Design review of the part built by this model. Coordinates are the model's own, in mm. A direction names the side the tool comes from. Give positions to 0.01 mm unless a question says otherwise; leave off trailing zeros. Order: outer loops, then holes, each group sorted by start corner. A loop starts at its lowest first (then second) coordinate and runs counter-clockwise, first axis right, second up.
Autodesk Inventor part; units mm, degrees
ref_plane "工作平面1" through (0, 0, 5.8) normal (0, 0, 1) x (1, 0, 0)
ref_plane "YZ Plane" through (0, 0, 0) normal (1, 0, 0) x (0, 1, 0)
ref_plane "XZ Plane" through (0, 0, 0) normal (0, 1, 0) x (-1, 0, 0)
sketch "草圖1" plane through (0, 0, 0) normal (0, 0, 1) x (1, 0, 0)
  circle A0 centre (0, 0) radius 26
  dimension "d0" = 52
extrude "擠出1" add sketch "草圖1" along normal blind 12.2
sketch "草圖2" plane through (0, 0, 12.2) normal (0, 0, 1) x (1, 0, 0)
  circle A0 centre (0, 0) radius 26
  circle A1 centre (0, 0) radius 20
  dimension "d3" = 40
extrude "擠出2" cut sketch "草圖2" against normal through all contours A1
sketch "草圖3" plane through (0, 0, 0) normal (0, 0, -1) x (-1, 0, 0)
  circle A0 centre (0, 0) radius 20
  circle A1 centre (0, 0) radius 26
  circle A2 centre (0, 0) radius 22.45
  dimension "d6" = 44.9
extrude "擠出3" cut sketch "草圖3" against normal blind 8.2 contours A2
ref_plane "工作平面1" through (0, 0, 5.8) normal (0, 0, 1) x (1, 0, 0)
sketch "草圖4" plane through (0, 0, 5.8) normal (0, 0, 1) x (1, 0, 0)
  circle A0 centre (0, 0) radius 24.4
  circle A1 centre (0, 0) radius 26
  dimension "d10" = 48.8
extrude "擠出4" cut sketch "草圖4" against normal blind 2.8
chamfer "倒角1" distance 0.4 angle 45 3 edges at (-26, 0, 12.2) (-26, 0, 0) (22.45, 0, 0)
chamfer "倒角2" distance 0.3 angle 45 1 edges at (-20, 0, 8.2)
properties part number "鑄鐵SLEEVE"
1. Take a section at A-A (y = 0). State the section outline as (x, z) points, then the cut area to 3 significant figures.
Recorded:
outline: (-26, 0.4) - (-25.6, 0) - (-22.85, 0) - (-22.45, 0.4) - (-22.45, 8.2) - (-20.3, 8.2) - (-20, 8.5) - (-20, 12.2) - (-25.6, 12.2) - (-26, 11.8) - (-26, 5.8) - (-24.4, 5.8) - (-24.4, 3) - (-26, 3) - close; (20, 8.5) - (20.3, 8.2) - (22.45, 8.2) - (22.45, 0.4) - (22.85, 0) - (25.6, 0) - (26, 0.4) - (26, 3) - (24.4, 3) - (24.4, 5.8) - (26, 5.8) - (26, 11.8) - (25.6, 12.2) - (20, 12.2) - close
area: 96.7 mm2
2. Take a section at D-D (z = 11). State the section outline as (x, y) points.
Recorded:
outline: circle Ø52 at (0, 0); hole circle Ø40 at (0, 0)
3. Machinability: for faces 1 (the face through (-20.633, 15.821, 8.758)), 2 (the face through (17, -12, 8.2)), which of the approach directions +Z, -Z, +X, -X, +Y, -Y give a long, thin tool a straight path to every point of the face, cutting with its end or side? Answer none if there is none.
Recorded:
face 1: +Z, -Z
face 2: -Z
4. For pin 1 (5 mm diameter, centred on y = -7.5, z = 4.5, fed in from +X); pin 2 (1.5 mm diameter, centred on y = 10, z = 4.5, fed in from +X); pin 3 (3 mm diameter, centred on x = 2.5, z = 8, fed in from -Y); pin 4 (15.5 mm diameter, centred on x = 9, y = -4, fed in from +Z), all flat-tipped, find the tip position at first contact; note any pin that passes through.
Recorded:
pin 1: stops at x = 25.44
pin 2: stops at x = 22.58
pin 3: stops at y = -25.98
pin 4: passes through
5. Draft analysis for pull direction Z (two halves, no side actions). For faces 3 (the face through (-15.3, 17.2, 0)), 4 (the face through (-4.336, -19.524, 10.376)), 5 (the face through (-24.376, 1.073, 4.42)), state which applies: pulls with the +Z half, pulls with the -Z half, needs draft (parallel to the pull), parting line crosses it, or undercut.
Recorded:
face 3: pulls with the -Z half
face 4: needs draft
face 5: undercut
6. Take a section at C-C (z = 6.75). State the section outline as (x, y) points.
Recorded:
outline: circle Ø52 at (0, 0); hole circle Ø44.9 at (0, 0)
7. For line 1 along Y through (x, z) = (0, 10); line 2 along Z through (x, y) = (-6, -24); line 3 along Y through (x, z) = (0, 5), list the stretches that pass through material, from the lowest coordinate up.
Recorded:
line 1: y = -26 to -20, 20 to 26
line 2: z = 0 to 3, 5.8 to 12.2
line 3: y = -24.4 to -22.45, 22.45 to 24.4
